The listing builds one solid part. Answer for the finished solid, in the listing's coordinates (mm). Give positions to 0.01 mm unless a question says otherwise; leave off trailing zeros. Write each loop counter-clockwise with the first axis right and the second up, starting at its lowest first coordinate (ties: lowest second). Pieces come first, ordered by that corner, then holes. Notation, with made-up numbers: M 32,60.5 L 90,60.5 A22 ccw 90,96.5 Z; hole C 84,-10 d2. An arc over 180 degrees is marked long. Answer as a JSON object with one key per item and string values.
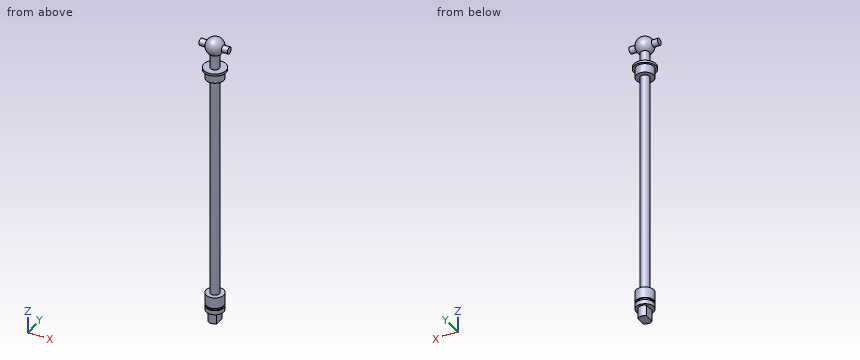
```python
from build123d import *

# Parameters (mm, degrees)
CUT_EXTRUDE1_DEPTH  = 5
SKETCH3_R           = 1.5
BOSS_EXTRUDE1_DEPTH = 6.5


with BuildPart() as part:
    # Sketch1 → Revolve1 (revolve)
    with BuildSketch(Plane(origin=(0, 0, 0), x_dir=(0, 0, -1), z_dir=(1, 0, 0))):
        with BuildLine():
            Line((7.464101615, 2), (14, 2))
            Line((14, 2), (14, 5))
            Line((14, 5), (15, 5))
            Line((15, 5), (15, 4))
            Line((15, 4), (19, 4))
            Line((19, 4), (19, 2))
            Line((19, 2), (121, 2))
            Line((121, 2), (121, 4))
            Line((121, 4), (126, 4))
            Line((126, 4), (126, 3.5))
            Line((126, 3.5), (127, 3.5))
            Line((127, 3.5), (127, 4))
            Line((127, 4), (129, 4))
            Line((129, 4), (129, 3))
            Line((129, 3), (134, 3))
            Line((134, 3), (134, 0))
            Line((134, 0), (0, 0))
            ThreePointArc((0, 0), (2.96472382, 3.863703305), (7.464101615, 2))
        make_face()
    revolve(axis=Axis((0, 0, 0), (0, 0, -1)))

    # Sketch2 → Cut-Extrude1 (cut)
    with BuildSketch(Plane(origin=(0, 0, -134), x_dir=(-1, 0, 0), z_dir=(0, 0, -1))):
        with BuildLine():
            ThreePointArc((-2, 2.236067977), (-3, 0), (-2, -2.236067977))
            Line((-2, -2.236067977), (-2, 2.236067977))
        make_face()
        with BuildLine():
            Line((2, 2.236067977), (2, -2.236067977))
            ThreePointArc((2, -2.236067977), (2.738612788, -1.224744871), (3, 0))
            ThreePointArc((3, 0), (2.738612788, 1.224744871), (2, 2.236067977))
        make_face()
    extrude(amount=-CUT_EXTRUDE1_DEPTH, mode=Mode.SUBTRACT)

    # Sketch3 → Boss-Extrude1 (add, symmetric)
    with BuildSketch(Plane(origin=(0, 0, 0), x_dir=(0, 0, -1), z_dir=(1, 0, 0))):
        with Locations((4, 0)):
            Circle(SKETCH3_R)
    extrude(amount=BOSS_EXTRUDE1_DEPTH, both=True)


solid = part.part
```
1. A cutting plane is placed at C-C, the plane z = -56. Give the vertices of the cut face in (x, y).
Verdict:
{"outline": "C 0,0 d4"}
2. Consider line 1 along Z through (x, y) = (-1, -2.5); line 2 along Z through (x, y) = (-0.75, -3.5); line 3 along Z through (x, y) = (3.25, -0.5). Determine where each line is inside the solid, lowest interval first.
Verdict:
{"line 1": "z = -134 to -121, -19 to -14, -6.96 to -1.04", "line 2": "z = -129 to -127, -126 to -121, -19 to -14, -5.79 to -2.21", "line 3": "z = -129 to -121, -19 to -14, -6.28 to -1.72"}
3. A cutting plane is placed at A-A, the plane z = -4. Give the vertices of the cut face in (x, y).
Verdict:
{"outline": "M -6.5,-1.5 L -3.71,-1.5 A4 ccw 3.71,-1.5 L 6.5,-1.5 L 6.5,1.5 L 3.71,1.5 A4 ccw -3.71,1.5 L -6.5,1.5 Z"}
4. Flat-ended cylindrical pins translate along their axes: pin 1 (4 mm diameter, centred on x = -2, y = -2.5, fed in from +Z); pin 2 (2 mm diameter, centred on x = 0.5, z = -109, fed in from -Y); pin 3 (3.5 mm diameter, centred on y = 0, z = -132, fed in from -X); pin 4 (2 mm diameter, centred on y = -4, z = -81, fed in from -X) (3 decimals). Find the tip coordinate at first contact, or state that the pin passes through.
Verdict:
{"pin 1": "stops at z = -0.18", "pin 2": "stops at y = -2", "pin 3": "stops at x = -2", "pin 4": "passes through"}
